Solid Edge part; units mm, degrees
sketch "Sketch1" plane through (0, 24.13, -19) normal (0, 0, -1) x (1, 0, 0)
  line L0 (-34.92, -26.03) -> (34.92, -26.03)
  line L1 (34.92, -26.03) -> (34.92, 26.03)
  line L2 (34.92, 26.03) -> (-34.92, 26.03)
  line L3 (-34.92, 26.03) -> (-34.92, -26.03)
extrude "Protrusion1" add sketch "Sketch1" against normal blind 2
sketch "Sketch2" plane through (-29.21, 44.45, -11.0875) normal (0, 0, -1) x (1, 0, 0)
  circle A0 centre (0, 0) radius 3.5
  circle A1 centre (58.42, 0) radius 3.5
extrude "ExtrudedProtrusion_2" add sketch "Sketch2" along normal up to next
sketch "Sketch3" plane through (0, 24.13, -19) normal (0, 0, -1) x (1, 0, 0)
  circle A0 centre (-29.21, -20.32) radius 1.5
  circle A1 centre (29.21, -20.32) radius 1.5
extrude "Cutout1" cut sketch "Sketch3" against normal up to next
sketch "Sketch4" plane through (0, 24.13, -19) normal (0, 0, -1) x (1, 0, 0)
  circle A0 centre (-29.21, -20.32) radius 3
  circle A1 centre (29.21, -20.32) radius 3.5
extrude "ExtrudedCutout_2" cut sketch "Sketch4" against normal blind 1.5
sketch "Sketch5" plane through (0, 24.13, -19) normal (0, 0, -1) x (1, 0, 0)
  line L0 (-8.42, -26.867) -> (8.92, -26.867)
  line L1 (8.92, -26.867) -> (8.92, -8.13)
  line L2 (8.92, -8.13) -> (-8.42, -8.13)
  line L3 (-8.42, -8.13) -> (-8.42, -26.867)
extrude "Cutout2" cut sketch "Sketch5" against normal through all
fillet "Round_1" radius 2 2 edges at (32.71, 44.45, -17) (-25.71, 44.45, -17)
The listing builds one solid part. Answer for the finished solid, in the listing's coordinates (mm). A direction names the side the tool comes from. Coordinates: 2 decimals unless noted, no trailing zeros. Write each loop counter-clockwise with the first axis right and the second up, starting at its lowest first coordinate (ties: lowest second). Pieces come first, ordered by that corner, then holes. Notation, with made-up numbers: (10, -27) - (40, -27) arc R34 cw to (40, 10) - close; hole circle Ø6 at (86, 27.25). An arc over 180 degrees is marked (long way). Return JSON: item names as keys, results as strings. Group by question number.
Q1. For a pull along Y with two mould halves and no side action, classify faces 5 (the flat face through (0, -1.9, -18)), 6 (the cylindrical face through (27.71, 44.38, -14.34)), 7 (the flat face through (0, 19, -17)) as +Y half, -Y half, draft (parallel to the pull), parting line (faces both ways), or undercut.
Q2. Which of the six approach directions +Z, -Z, +X, -X, +Y, -Y give full straight-line access (tool end or side, diameter ignored) to faces 1 (the cylindrical face through (-32.207, 44.318, -18.26)), 2 (the cylindrical face through (-31.987, 42.32, -13.016)), 3 (the flat face through (-8.42, 41, -18)), 4 (the flat face through (34.92, 24, -18))?
Q3. The part is cut by section D-D on y = 44.45. State how many separate pieces and enclosed holes the cut face has, and give its area (3 significant figures).
Q4. The part is cut by section B-B on z = -12.5. Write down the section's boundary in (x, y), and give its area (3 significant figures).
Q5. Find the intervals of material crossed by line 1 along X through (y, z) = (44.45, -18.3); line 2 along Y through (x, z) = (29.21, -13); line 3 along Y through (x, z) = (29.21, -18.5), in increasing order. Write a range as [from, to].
Q6. Flat-ended cylindrical pins translate along their axes: pin 1 Ø0.6 at (x, z) = (-3, -18) entering from +Y; pin 2 Ø3.5 at (x, y) = (-29.21, 44.45) entering from -Z; pin 3 Ø4 at (x, y) = (-10, 28.5) entering from +Z. Find the tip coordinate at first contact, or state that the pin passes through.
Q7. The part is cut by section A-A on x = -29.21. Write down the section's boundary in (y, z).
Q8. The part is cut by section C-C on x = 29.21. Write down the section's boundary in (y, z), and give its area (3 significant figures).
Evaluation:
{
 "1": {"face 5": "-Y half", "face 6": "undercut", "face 7": "draft"},
 "2": {"face 1": "-Z", "face 2": "+Z", "face 3": "+Z, -Z, +Y", "face 4": "+Z, -Z, +X, +Y, -Y"},
 "3": {"separate pieces": "4", "enclosed holes": "0", "area": "133 mm2"},
 "4": {"outline": "circle Ø7 at (-29.21, 44.45); circle Ø7 at (29.21, 44.45); hole circle Ø3 at (-29.21, 44.45); hole circle Ø3 at (29.21, 44.45)", "area": "62.8 mm2"},
 "5": {"line 1": "x = [-34.92, -32.21], [-26.21, -8.42], [8.92, 25.71], [32.71, 34.92]", "line 2": "y = [40.95, 42.95], [45.95, 47.95]", "line 3": "y = [-1.9, 40.95], [47.95, 50.16]"},
 "6": {"pin 1": "stops at y = 32.26", "pin 2": "stops at z = -17.5", "pin 3": "stops at z = -17"},
 "7": {"outline": "(-1.9, -19) - (41.45, -19) - (41.45, -17.5) - (42.95, -17.5) - (42.95, -11.09) - (40.95, -11.09) - (40.95, -15) arc R2 cw to (38.95, -17) - (-1.9, -17) - close; (45.95, -17.5) - (47.45, -17.5) - (47.45, -19) - (50.16, -19) - (50.16, -17) - (49.95, -17) arc R2 cw to (47.95, -15) - (47.95, -11.09) - (45.95, -11.09) - close"},
 "8": {"outline": "(-1.9, -19) - (40.95, -19) - (40.95, -17.5) - (42.95, -17.5) - (42.95, -11.09) - (40.95, -11.09) - (40.95, -15) arc R2 cw to (38.95, -17) - (-1.9, -17) - close; (45.95, -17.5) - (47.95, -17.5) - (47.95, -19) - (50.16, -19) - (50.16, -17) - (49.95, -17) arc R2 cw to (47.95, -15) - (47.95, -11.09) - (45.95, -11.09) - close", "area": "117 mm2"}
}
